from build123d import *

# Parameters (mm, degrees)
BOSS_EXTRUDE1_DEPTH      = 3
BOSS_EXTRUDE1_DEPTH_BACK = 3
SKETCH1_R                = 1.5
SKETCH2_W                = 5
SKETCH2_H                = 52.625164332
BOSS_EXTRUDE2_DEPTH      = 5
SKETCH3_W                = 26.14370814
SKETCH3_H                = 16.696493178
BOSS_EXTRUDE3_DEPTH      = 13
SKETCH4_W                = 9.938286277
SKETCH4_H                = 10.344826846
BOSS_EXTRUDE4_DEPTH      = 6
SKETCH5_W                = 12.473423639
SKETCH5_H                = 10.432804083
BOSS_EXTRUDE5_DEPTH      = 13
SKETCH6_W                = 21.73915334
SKETCH6_H                = 8.30143682
BOSS_EXTRUDE6_DEPTH      = 6


with BuildPart() as part:
    # Sketch1 → Boss-Extrude1 (new, two sides: drawn at the far end of the back side and taken through both)
    with BuildSketch(Plane(origin=(0, 0, 0), x_dir=(1, 0, 0), z_dir=(0, 1, 0)).offset(-BOSS_EXTRUDE1_DEPTH_BACK)):
        with BuildLine():
            Line((-39.5, -30), (39.5, -30))
            ThreePointArc((39.5, -30), (41.621320344, -29.121320344), (42.5, -27))
            Line((42.5, -27), (42.5, 27))
            ThreePointArc((42.5, 27), (41.621320344, 29.121320344), (39.5, 30))
            Line((39.5, 30), (-39.5, 30))
            ThreePointArc((-39.5, 30), (-41.621320344, 29.121320344), (-42.5, 27))
            Line((-42.5, 27), (-42.5, -27))
            ThreePointArc((-42.5, -27), (-41.621320344, -29.121320344), (-39.5, -30))
        make_face()
        with Locations(Location((-39.5, 27, 0), (0, 0, 270))):
            Circle(SKETCH1_R, mode=Mode.SUBTRACT)
        with Locations(Location((39.5, 27, 0), (0, 0, 270))):
            Circle(SKETCH1_R, mode=Mode.SUBTRACT)
        with Locations(Location((39.5, -27, 0), (0, 0, 270))):
            Circle(SKETCH1_R, mode=Mode.SUBTRACT)
        with Locations(Location((-39.5, -27, 0), (0, 0, 270))):
            Circle(SKETCH1_R, mode=Mode.SUBTRACT)
    extrude(amount=BOSS_EXTRUDE1_DEPTH + BOSS_EXTRUDE1_DEPTH_BACK)

    # Sketch2 → Boss-Extrude2 (add)
    with BuildSketch(Plane(origin=(0, 0, 0), x_dir=(1, 0, 0), z_dir=(0, 1, 0))):
        with Locations((-33.860518443, 0)):
            Rectangle(SKETCH2_W, SKETCH2_H)
    extrude(amount=BOSS_EXTRUDE2_DEPTH)

    # Sketch3 → Boss-Extrude3 (add)
    with BuildSketch(Plane(origin=(0, 0, 0), x_dir=(1, 0, 0), z_dir=(0, 1, 0))):
        with Locations((29.42814593, 12.489663364)):
            Rectangle(SKETCH3_W, SKETCH3_H)
    extrude(amount=BOSS_EXTRUDE3_DEPTH)

    # Sketch4 → Boss-Extrude4 (add)
    with BuildSketch(Plane(origin=(0, 0, 0), x_dir=(1, 0, 0), z_dir=(0, 1, 0))):
        with Locations((37.530856861, -4.519547668)):
            Rectangle(SKETCH4_W, SKETCH4_H)
    extrude(amount=BOSS_EXTRUDE4_DEPTH)

    # Sketch5 → Boss-Extrude5 (add)
    with BuildSketch(Plane(origin=(0, 0, 0), x_dir=(1, 0, 0), z_dir=(0, 1, 0))):
        with Locations((7.14417266, -22.535803866)):
            Rectangle(SKETCH5_W, SKETCH5_H)
    extrude(amount=BOSS_EXTRUDE5_DEPTH)

    # Sketch6 → Boss-Extrude6 (add)
    with BuildSketch(Plane(origin=(0, 0, 0), x_dir=(1, 0, 0), z_dir=(0, 1, 0))):
        with Locations((26.117763778, -22.537195349)):
            Rectangle(SKETCH6_W, SKETCH6_H)
    extrude(amount=BOSS_EXTRUDE6_DEPTH)


solid = part.part
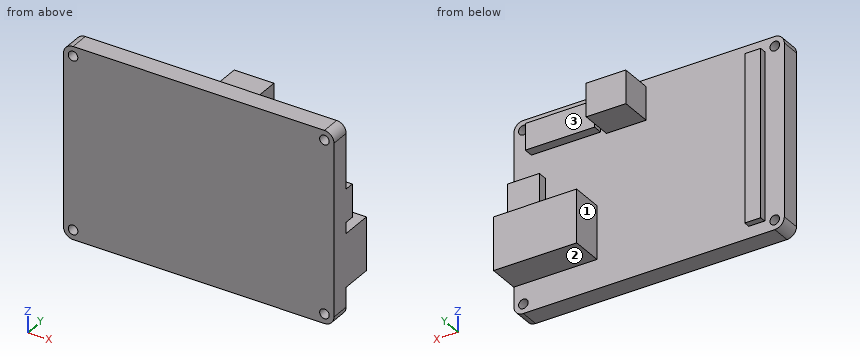
Geometry check sheet. Reference: the model listing, model coordinates, mm. Face numbers are marked on the shaded views. A direction names the side the tool comes from. Round coordinates to 2 decimals unless told otherwise and drop trailing zeros. Loops run counter-clockwise (first coordinate to the right, second up) from the corner with the lowest first, then second, coordinate; pieces in that order, holes last. Notation, with made-up numbers: (25.5, 39.5) - (81.5, 39.5) arc R21 cw to (81.5, 54.5) - close; hole circle Ø11 at (41.5, -1.5). An arc over 180 degrees is marked (long way). Answer as CSV lines item,"result".
(1) Cross-section at C-C, the plane z = 21.5. Enter the section's corners in (x, y).
Output values:
outline,"(-42.5, -3) - (42.5, -3) - (42.5, 3) - (36.99, 3) - (36.99, 6) - (15.25, 6) - (15.25, 3) - (13.38, 3) - (13.38, 13) - (0.91, 13) - (0.91, 3) - (-31.36, 3) - (-31.36, 5) - (-36.36, 5) - (-36.36, 3) - (-42.5, 3) - close"
(2) Depth check by flat-ended pin: pin 1 Ø3.5 at (x, y) = (38.5, 4) entering from -Z; pin 2 Ø8 at (x, z) = (40, 2) entering from +Y; pin 3 Ø3 at (x, y) = (24, 6.5) entering from -Z; pin 4 Ø2.5 at (x, y) = (28, 4.5) entering from +Z. Enter the tip coordinate at first touch or a pass-through.
Output values:
pin 1,"stops at z = -30"
pin 2,"stops at y = 6"
pin 3,"stops at z = -20.84"
pin 4,"stops at z = 26.69"
(3) Set-up check for the marked faces 1, 2 and 3: record each of +Z, -Z, +X, -X, +Y, -Y from which the full face is reachable in a straight line by a thin tool's end or side.
Output values:
face 1,"-Z, +Y"
face 2,"-Z, +X, +Y"
face 3,"+Z, +X, +Y"
(4) Cross-section at A-A, the plane y = 4. Enter the section's corners in (x, z), and give its area (3 significant figures).
Output values:
outline,"(-36.36, -26.31) - (-31.36, -26.31) - (-31.36, 26.31) - (-36.36, 26.31) - close; (0.91, 17.32) - (13.38, 17.32) - (13.38, 27.75) - (0.91, 27.75) - close; (15.25, 18.39) - (36.99, 18.39) - (36.99, 26.69) - (15.25, 26.69) - close; (16.36, -20.84) - (42.5, -20.84) - (42.5, -4.14) - (16.36, -4.14) - close; (32.56, -0.65) - (42.5, -0.65) - (42.5, 9.69) - (32.56, 9.69) - close"
area,"1,110 mm²"
(5) Material ranges on line 1 along X through (y, z) = (0.35, -27); line 2 along X through (y, z) = (4.75, -12); line 3 along X through (y, z) = (5.5, 20), recorded low to high.
Output values:
line 1,"x = -42.5 to -41, -38 to 38, 41 to 42.5"
line 2,"x = -36.36 to -31.36, 16.36 to 42.5"
line 3,"x = 0.91 to 13.38, 15.25 to 36.99"
(6) Cross-section at B-B, the plane y = 11.25. Enter the section's corners in (x, z).
Output values:
outline,"(0.91, 17.32) - (13.38, 17.32) - (13.38, 27.75) - (0.91, 27.75) - close; (16.36, -20.84) - (42.5, -20.84) - (42.5, -4.14) - (16.36, -4.14) - close"
(7) Cross-section at D-D, the plane z = -15. Enter the section's corners in (x, y).
Output values:
outline,"(-42.5, -3) - (42.5, -3) - (42.5, 13) - (16.36, 13) - (16.36, 3) - (-31.36, 3) - (-31.36, 5) - (-36.36, 5) - (-36.36, 3) - (-42.5, 3) - close"
